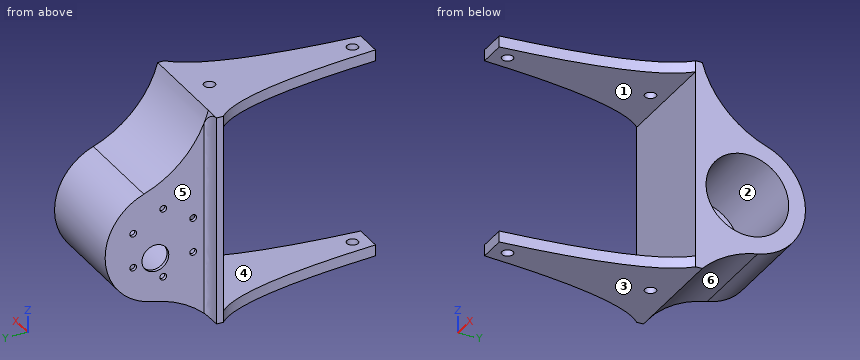
from build123d import *

# Parameters (mm, degrees)
BOSS_EXTRUDE1_DEPTH      = 5
BOSS_EXTRUDE2_START      = -84
BOSS_EXTRUDE2_DEPTH      = 5
BOSS_EXTRUDE7_DEPTH      = 21
BOSS_EXTRUDE7_DEPTH_BACK = 29
BOSS_EXTRUDE7_START      = 4
SKETCH9_W                = 94
SKETCH9_H                = 3
CUT_EXTRUDE1_DEPTH       = 106.948100654
CUT_EXTRUDE1_DEPTH_BACK  = 106.948100654
SKETCH5_R                = 2.5
BOSS_EXTRUDE9_START      = -8.5
SKETCH13_R               = 18.5
BOSS_EXTRUDE9_DEPTH      = 41.5
BOSS_EXTRUDE10_START     = 1.5
SKETCH15_R               = 1.5
SKETCH15_R_2             = 6
BOSS_EXTRUDE10_DEPTH     = 1.5
FILLET2_R                = 46
FILLET4_SIZE             = 2
FILLET4_SIZE_2           = 7


with BuildPart() as part:
    # Sketch2 → Boss-Extrude1 (new body)
    with BuildSketch(Plane.XY):
        with BuildLine():
            Line((6.25, -39), (-6.25, -39))
            add(Edge.make_bspline(
                [(-25, 39), (-10.900418278, 25.328341358), (-6.25, -39)],
                knots=[0, 0, 0, 1, 1, 1], degree=2))
            Line((-25, 39), (25, 39))
            add(Edge.make_bspline(
                [(25, 39), (10.900418278, 25.328341358), (6.25, -39)],
                knots=[0, 0, 0, 1, 1, 1], degree=2))
        make_face()
    extrude(amount=BOSS_EXTRUDE1_DEPTH)



with BuildPart() as body_2:
    # Sketch3 → Boss-Extrude2 (new body)
    with BuildSketch(Plane.XY.offset(BOSS_EXTRUDE2_START)):
        with BuildLine():
            Line((6.25, -39), (-6.25, -39))
            add(Edge.make_bspline(
                [(-25, 39), (-10.900418278, 25.328341358), (-6.25, -39)],
                knots=[0, 0, 0, 1, 1, 1], degree=2))
            Line((-25, 39), (25, 39))
            add(Edge.make_bspline(
                [(25, 39), (10.900418278, 25.328341358), (6.25, -39)],
                knots=[0, 0, 0, 1, 1, 1], degree=2))
        make_face()
    extrude(amount=-BOSS_EXTRUDE2_DEPTH)


with BuildPart() as part_1:
    add(part.part)

    add(body_2.part)  # Boss-Extrude7 merges body 2
    # Sketch9 → Boss-Extrude7 (add, two sides: drawn at the far end of the back side and taken through both)
    with BuildSketch(Plane(origin=(0, 0, 0), x_dir=(0, 0, -1), z_dir=(1, 0, 0)).offset(BOSS_EXTRUDE7_START - BOSS_EXTRUDE7_DEPTH_BACK)):
        with Locations((42, 40.5)):
            Rectangle(SKETCH9_W, SKETCH9_H)
    extrude(amount=BOSS_EXTRUDE7_DEPTH + BOSS_EXTRUDE7_DEPTH_BACK)

    # Sketch5 → Cut-Extrude1 (cut, two sides: drawn at the far end of the back side and taken through both)
    with BuildSketch(Plane.XY.offset(5).offset(-CUT_EXTRUDE1_DEPTH_BACK)):
        with Locations((0, 32)):
            Circle(SKETCH5_R)
        with Locations((0, -32)):
            Circle(SKETCH5_R)
    extrude(amount=CUT_EXTRUDE1_DEPTH + CUT_EXTRUDE1_DEPTH_BACK, mode=Mode.SUBTRACT)

    # Sketch13 → Boss-Extrude9 (add)
    with BuildSketch(Plane.ZY.offset(25).offset(BOSS_EXTRUDE9_START)):
        with BuildLine():
            Line((-66.479483804, 42), (-33.740516196, 42))
            ThreePointArc((-33.740516196, 42), (-50.11, 88.2), (-66.479483804, 42))
        make_face()
        with Locations(Location((-50.11, 62.2, 0), (0, 0, 180))):
            Circle(SKETCH13_R, mode=Mode.SUBTRACT)
    extrude(amount=-BOSS_EXTRUDE9_DEPTH)

    # Sketch15 → Boss-Extrude10 (add)
    with BuildSketch(Plane.ZY.offset(16.5).offset(BOSS_EXTRUDE10_START)):
        with BuildLine():
            Line((-66.479483804, 42), (-33.740516196, 42))
            ThreePointArc((-33.740516196, 42), (-50.11, 88.2), (-66.479483804, 42))
        make_face()
        with Locations((-34.61, 62.2)):
            Circle(SKETCH15_R, mode=Mode.SUBTRACT)
        with Locations((-42.36, 48.776606241)):
            Circle(SKETCH15_R, mode=Mode.SUBTRACT)
        with Locations((-57.86, 48.776606241)):
            Circle(SKETCH15_R, mode=Mode.SUBTRACT)
        with Locations((-65.61, 62.2)):
            Circle(SKETCH15_R, mode=Mode.SUBTRACT)
        with Locations((-57.86, 75.623393759)):
            Circle(SKETCH15_R, mode=Mode.SUBTRACT)
        with Locations((-42.36, 75.623393759)):
            Circle(SKETCH15_R, mode=Mode.SUBTRACT)
        with Locations((-56.172177826, 65.7)):
            Circle(SKETCH15_R_2, mode=Mode.SUBTRACT)
    extrude(amount=-BOSS_EXTRUDE10_DEPTH)

    # Fillet2
    # the kernel refuses this fillet: 46 mm, written as the material it adds along each edge
    with BuildSketch(Plane(origin=(-18, 42, -66.479483804), x_dir=(0, 0, -1), z_dir=(1, 0, 0))) as fillet2_piece_1:
        with BuildLine():
            CenterArc((54.465764785, 33.098354832), FILLET2_R, 190.319893555, 35.695751296)
            Line((9.20991152, 24.857739245), (8.304794455, 24.692926933))
            ThreePointArc((8.304794455, 24.692926933), (7.148225336, 11.486576056), (-0.579227888, 0.714769231))
            Line((-0.579227888, 0.714769231), (0, -0.92))
            ThreePointArc((0, -0.92), (11.260258098, -0.92), (21.881611225, -0.661967097))
            Line((21.881611225, -0.661967097), (22.520516196, 0))
        make_face()
    extrude(amount=43)
    with BuildSketch(Plane(origin=(25, 42, -33.740516196), x_dir=(0, 0, 1), z_dir=(-1, 0, 0))) as fillet2_piece_2:
        with BuildLine():
            CenterArc((51.516198575, 44.19029237), FILLET2_R, 199.46302715, 54.412069486)
            Line((8.144790389, 28.863161134), (7.277362225, 28.556618509))
            ThreePointArc((7.277362225, 28.556618509), (7.767902037, 13.388758941), (-0.579227888, 0.714769231))
            Line((-0.579227888, 0.714769231), (0, -0.92))
            ThreePointArc((0, -0.92), (19.370258098, -0.92), (38.485002549, -0.883805847))
            Line((38.485002549, -0.883805847), (38.740516196, 0))
        make_face()
    extrude(amount=43)

    # Fillet4
    # an asymmetric fillet: 7, 2 mm, written as the material it adds along each edge
    with BuildSketch(Plane(origin=(-18, 42, -89), x_dir=(0, 1, 0), z_dir=(0, 0, 1))) as fillet4_piece_1_section:
        with BuildLine():
            Bezier((FILLET4_SIZE, 0), (0, 0), (0, FILLET4_SIZE_2), weights=[1, 0.707106781, 1])
            Line((0, FILLET4_SIZE_2), (0, 0))
            Line((0, 0), (FILLET4_SIZE, 0))
        make_face()
    fillet4_piece_1 = extrude(amount=94, mode=Mode.PRIVATE)
    fillet4_piece_1 = fillet4_piece_1 - Plane(origin=(-19.911254264, 86.19029237, 17.775682378), x_dir=(0, 0, 1), z_dir=(1, 0, 0)) * Cylinder(46, 216, mode=Mode.PRIVATE)
    fillet4_piece_1 = fillet4_piece_1 - Plane(origin=(-19.911254264, 75.098354832, -120.945248589), x_dir=(0, 0, -1), z_dir=(-1, 0, 0)) * Cylinder(46, 216, mode=Mode.PRIVATE)
    add(fillet4_piece_1)


solid = part_1.part
Design review of the part built by this model. Coordinates are the model's own, in mm. Face numbers are marked on the shaded views. A direction names the side the tool comes from. Coordinates: 2 decimals unless noted, no trailing zeros. Write each loop counter-clockwise with the first axis right and the second up, starting at its lowest first coordinate (ties: lowest second). Pieces come first, ordered by that corner, then holes. Notation, with made-up numbers: (8, 18) -> (34, 18) arc R12 ccw to (34, 40) -> close; hole circle Ø7 at (-30, 32.25). An arc over 180 degrees is marked (long way). Write each question's results on one line, items separated by ' | '. Start each with the question number.
(1) Take a section at A-A on x = 0. Write out the cut boundary in (y, z), and give its area (3 significant figures).
(2) Take a section at C-C on y = 53.5. Write out the cut boundary in (x, z).
(3) Tool access review of the marked faces 1, 2 and 3: name each direction out of +Z, -Z, +X, -X, +Y, -Y from which nothing blocks a thin tool from reaching the whole face with its end or side.
(4) The part is to be moulded in two halves that separate along Z. For the marked faces 4, 5 and 6, say which applies: pulls with the +Z half, pulls with the -Z half, needs draft (parallel to the pull), parting line crosses it, or undercut.
(5) For line 1 along Z through (x, y) = (7, 16); line 2 along Y through (x, z) = (-17, -57); line 3 along Y through (x, z) = (0, 1), list the stretches that pass through material, from the lowest coordinate up. Write a range as from..to.
(6) Clearance check with flat-ended pins moving along their axes: P1, Ø14, axis at y = 65.7, z = -56.17, coming from the +X side; P2, Ø8, axis at x = -14.5, y = 69.5, coming from the -Z side; P3, Ø2, axis at x = 3, z = -35.5, coming from the -Y side; P4, Ø1.8, axis at y = 48.78, z = -57.86, coming from the +X side. State where each tip first meets the part, or that it passes through.
(7) Take a section at B-B on y = 32. Give the number of separate pieces and of enclosed holes in the cut face, and give its area (3 significant figures).
Results found:
1) outline: (-39, -89) -> (-34.5, -89) -> (-34.5, -84) -> (-39, -84) -> close; (-39, 0) -> (-34.5, 0) -> (-34.5, 5) -> (-39, 5) -> close; (-29.5, -89) -> (29.5, -89) -> (29.5, -84) -> (-29.5, -84) -> close; (-29.5, 0) -> (29.5, 0) -> (29.5, 5) -> (-29.5, 5) -> close; (34.5, -89) -> (42, -89) arc R46 cw to (66.86, -75.69) arc R26 ccw to (70.86, -25.6) arc R46 cw to (42, 5) -> (34.5, 5) -> (34.5, 0) -> (39, 0) -> (39, -84) -> (34.5, -84) -> close; hole circle Ø37 at (62.2, -50.11) | area: 2,370 mm2
2) outline: (-18, -80.33) -> (25, -80.33) -> (25, -66.44) -> (-16.5, -66.44) -> (-16.5, -33.78) -> (25, -33.78) -> (25, -14.59) -> (-18, -14.59) -> close
3) face 1: +X, -X, -Y | face 2: +X | face 3: -Z, +X, -X, +Y, -Y
4) face 4: undercut | face 5: needs draft | face 6: pulls with the -Z half
5) line 1: z = -89..-84, 0..5 | line 2: y = 39..47.55, 50.01..59.76, 71.64..74.39, 76.85..87.27 | line 3: y = -39..-34.5, -29.5..29.5, 34.5..43.36
6) P1: stops at x = -16.5 | P2: stops at z = -75.96 | P3: stops at y = 39 | P4: passes through
7) separate pieces: 4 | enclosed holes: 0 | area: 350 mm2
